Part print with two shaded views. Sizes in mm from the minimum x, y, z corner. A direction names the side the tool comes from. Round coordinates to 2 decimals unless told otherwise and drop trailing zeros. Write each loop counter-clockwise with the first axis right and the second up, starting at its lowest first coordinate (ties: lowest second). Pieces come first, ordered by that corner, then holes. Notation, with made-up numbers: (21.25, 72.5) -> (29.25, 72.5) arc R28 ccw to (29.25, 111.5) -> close; hole circle Ø2 at (76, 50.5). An arc over 180 degrees is marked (long way). Answer as CSV lines item,"result".
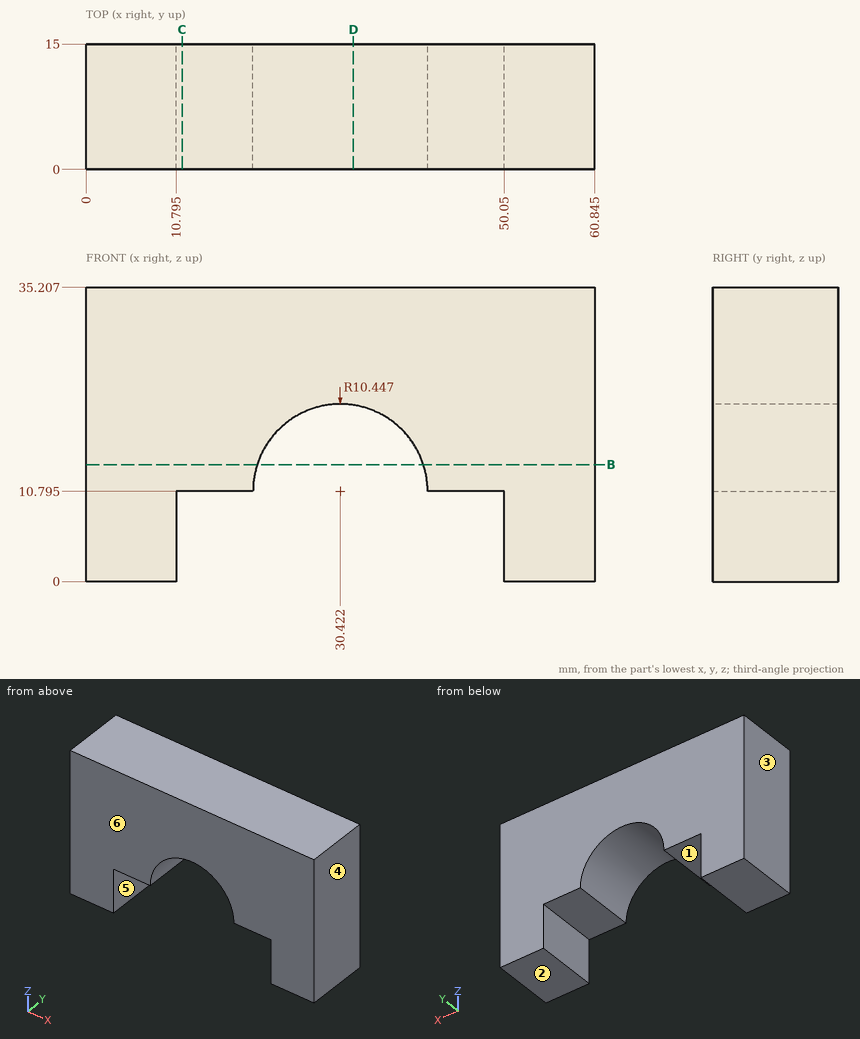
1. Cut at D-D, the plane x = 32. Write the cut outline in (y, z).
Results found:
outline,"(0, 21.12) -> (15, 21.12) -> (15, 35.21) -> (0, 35.21) -> close"
2. Drop flat-ended pins along their axis: pin 1 Ø2 at (x, y) = (7, 3) entering from -Z; pin 2 Ø7.5 at (x, y) = (17.5, 5.5) entering from -Z (1 decimal). Give the stop position or say it passes through.
Results found:
pin 1,"stops at z = 0"
pin 2,"stops at z = 10.8"
3. Cut at B-B, the plane z = 14. Write the cut outline in (x, y) (1 decimal).
Results found:
outline,"(0, 0) -> (20.5, 0) -> (20.5, 15) -> (0, 15) -> close; (40.4, 0) -> (60.8, 0) -> (60.8, 15) -> (40.4, 15) -> close"
4. Cut at C-C, the plane x = 11.5. Write the cut outline in (y, z) (1 decimal), then the cut area to 3 significant figures.
Results found:
outline,"(0, 10.8) -> (15, 10.8) -> (15, 35.2) -> (0, 35.2) -> close"
area,"366 mm2"
5. Mould opens along X. For the marked faces 3, 4, 5 and 6 say: +X half, -X half, draft (parallel to the pull), parting line (faces both ways), or undercut.
Results found:
face 3,"-X half"
face 4,"+X half"
face 5,"undercut"
face 6,"draft"
6. Probe line 1 along X through (y, z) = (13.75, 11) (1 decimal); line 2 along X through (y, z) = (3, 18.5) (1 decimal); line 3 along Z through (x, y) = (49, 10.25) (1 decimal). List the from-to ranges inside material, lowest first.
Results found:
line 1,"x = 0 to 20, 40.9 to 60.8"
line 2,"x = 0 to 23.4, 37.5 to 60.8"
line 3,"z = 10.8 to 35.2"
7. Which spindle directions (+Z, -Z, +X, -X, +Y, -Y) get a long thin tool onto all of the face, cutting with end or side? Do the marked faces 1 and 2. Say none if no direction does.
Results found:
face 1,"-Z, +Y, -Y"
face 2,"-Z, +X, -X, +Y, -Y"
